```python
from build123d import *

# Parameters (mm, degrees)
SKETCH1_W          = 153.56078
SKETCH1_H          = 114.3
SKETCH1_R          = 2.413
BASE_FLANGE1_DEPTH = 2.38125
FILLET1_R          = 6.35
SKETCH7_W          = 19.05
SKETCH7_H          = 114.3
CUT_EXTRUDE2_DEPTH = 2.54
FILLET2_R          = 6.35


# Sheet-metal steps are written as plain solids
with BuildPart() as part:
    # Sketch1 → Base-Flange1 (new body)
    with BuildSketch(Plane(origin=(0, 0, 0), x_dir=(1, 0, 0), z_dir=(0, 1, 0))):
        Rectangle(SKETCH1_W, SKETCH1_H)
        with Locations(Location((-63.5, -51.59375, 0), (0, 0, 270))):
            Circle(SKETCH1_R, mode=Mode.SUBTRACT)
        with Locations(Location((-38.1, -51.59375, 0), (0, 0, 270))):
            Circle(SKETCH1_R, mode=Mode.SUBTRACT)
        with Locations(Location((-12.7, -51.59375, 0), (0, 0, 270))):
            Circle(SKETCH1_R, mode=Mode.SUBTRACT)
        with Locations(Location((12.7, -51.59375, 0), (0, 0, 270))):
            Circle(SKETCH1_R, mode=Mode.SUBTRACT)
        with Locations(Location((38.1, -51.59375, 0), (0, 0, 270))):
            Circle(SKETCH1_R, mode=Mode.SUBTRACT)
        with Locations(Location((63.5, -51.59375, 0), (0, 0, 270))):
            Circle(SKETCH1_R, mode=Mode.SUBTRACT)
        with Locations(Location((63.5, 51.59375, 0), (0, 0, 270))):
            Circle(SKETCH1_R, mode=Mode.SUBTRACT)
        with Locations(Location((38.1, 51.59375, 0), (0, 0, 270))):
            Circle(SKETCH1_R, mode=Mode.SUBTRACT)
        with Locations(Location((12.7, 51.59375, 0), (0, 0, 270))):
            Circle(SKETCH1_R, mode=Mode.SUBTRACT)
        with Locations(Location((-12.7, 51.59375, 0), (0, 0, 270))):
            Circle(SKETCH1_R, mode=Mode.SUBTRACT)
        with Locations(Location((-38.1, 51.59375, 0), (0, 0, 270))):
            Circle(SKETCH1_R, mode=Mode.SUBTRACT)
        with Locations(Location((-63.5, 51.59375, 0), (0, 0, 270))):
            Circle(SKETCH1_R, mode=Mode.SUBTRACT)
        Polygon((57.73039, -41.275), (-63.104482091, -41.275), (-63.104482091, 41.275), (21.327886111, 41.275), (57.73039, 41.275), (57.73039, 15.875), align=None, mode=Mode.SUBTRACT)
    extrude(amount=-BASE_FLANGE1_DEPTH)

    # Fillet1
    fillet1_edges = [part.edges().sort_by_distance(p)[0] for p in [
        (-76.78039, -1.190625, -57.15),
        (76.78039, -1.190625, -57.15),
        (76.78039, -1.190625, 57.15),
        (-76.78039, -1.190625, 57.15),
    ]]
    fillet(fillet1_edges, radius=FILLET1_R)

    # Sketch7 → Cut-Extrude2 (cut)
    with BuildSketch(Plane(origin=(0, -2.38125, 0), x_dir=(-1, 0, 0), z_dir=(0, -1, 0))):
        with Locations((67.25539, 0)):
            Rectangle(SKETCH7_W, SKETCH7_H)
    extrude(amount=-CUT_EXTRUDE2_DEPTH, mode=Mode.SUBTRACT)

    # Fillet2
    fillet2_edges = [part.edges().sort_by_distance(p)[0] for p in [
        (-57.73039, -1.190625, 41.275),
        (-57.73039, -1.190625, -41.275),
        (-57.73039, -1.190625, 57.15),
        (-57.73039, -1.190625, -57.15),
    ]]
    fillet(fillet2_edges, radius=FILLET2_R)


solid = part.part
```
Design review of the part built by this model. Coordinates are the model's own, in mm. A direction names the side the tool comes from. Round coordinates to 2 decimals unless told otherwise and drop trailing zeros. Order: outer loops, then holes, each group sorted by start corner. A loop starts at its lowest first (then second) coordinate and runs counter-clockwise, first axis right, second up. Notation, with made-up numbers: M 33,0 L 75,0 A14 ccw 75,16 Z; hole C 53.25,50 d9. An arc over 180 degrees is marked long. Put each result on its own line as item: value.
Q1. Draft analysis for pull direction Z (two halves, no side actions). For faces 1 (the face through (-13.624, -1.174, 53.823)), 2 (the face through (59, -2.381, 0)), 3 (the face through (74.97, -1.21, -55.24)), state which applies: released by +Z, released by -Z, zero draft, split by the parting line, or undercut.
Reported:
face 1: undercut
face 2: zero draft
face 3: released by -Z
Q2. Insertion check: pin 1 Ø1.2 at (y, z) = (-1, -3.5) entering from -X. The pin has a flat end and moves straight along its axis. Give the tip position at first contact, or say it passes through.
Reported:
pin 1: x = 57.73
Q3. To check wall thickness, follow line 1 (Z direction, x = 52.5, y = -1.9) (3 decimals); line 2 (Z direction, x = 13, y = -1.6) (3 decimals); line 3 (Z direction, x = 64, y = -1.6). State the ranges of each line that lie inside material, in increasing order.
Reported:
line 1: -57.15 to -41.275, 41.275 to 57.15
line 2: -57.15 to -53.988, -49.199 to -41.275, 41.275 to 49.199, 53.988 to 57.15
line 3: -57.15 to -53.95, -49.23 to 49.23, 53.95 to 57.15
Q4. Machinability: for faces 4 (the face through (-39.024, -1.174, -49.365)), 5 (the face through (-55.92, -1.174, 43.185)), which of the approach directions +Z, -Z, +X, -X, +Y, -Y give a long, thin tool a straight path to every point of the face, cutting with its end or side? Answer none if there is none.
Reported:
face 4: +Y, -Y
face 5: -X, +Y, -Y
Q5. Consider section A-A (x = -5). State the section outline as (y, z) points (3 decimals), and give its area (3 significant figures).
Reported:
outline: M -2.381,-57.15 L 0,-57.15 L 0,-41.275 L -2.381,-41.275 Z; M -2.381,41.275 L 0,41.275 L 0,57.15 L -2.381,57.15 Z
area: 75.6 mm²
Q6. Consider section D-D (z = -24). State the section outline as (x, y) points.
Reported:
outline: M 57.73,-2.38 L 76.78,-2.38 L 76.78,0 L 57.73,0 Z
Q7. Consider section C-C (y = -0.6). State how many separate pieces and enclosed holes the cut face has, and give its area (3 significant figures).
Reported:
separate pieces: 1
enclosed holes: 10
area: 5,610 mm²
Q8. Consider section B-B (x = 38.1). State the section outline as (y, z) points (3 decimals).
Reported:
outline: M -2.381,-57.15 L 0,-57.15 L 0,-54.007 L -2.381,-54.007 Z; M -2.381,-49.181 L 0,-49.181 L 0,-41.275 L -2.381,-41.275 Z; M -2.381,41.275 L 0,41.275 L 0,49.181 L -2.381,49.181 Z; M -2.381,54.007 L 0,54.007 L 0,57.15 L -2.381,57.15 Z
